Read the model definition and answer for the solid it produces. Units are mm, in the model's axes. A direction names the side the tool comes from. Coordinates: 2 decimals unless noted, no trailing zeros. Order: outer loops, then holes, each group sorted by start corner. A loop starts at its lowest first (then second) coordinate and runs counter-clockwise, first axis right, second up. Notation, with made-up numbers: (11, 1.5) -> (23, 1.5) arc R24 ccw to (23, 30.5) -> close; hole circle Ø7 at (-18.75, -36). An arc over 180 degrees is marked (long way). Use CSV: the item, a comma, the result in double quotes.
```python
from build123d import *

# Parameters (mm, degrees)
F1_ANGLE = 180
F2_R     = 18
F2_R_2   = 4.0025
F3_DEPTH = 14
F5_R     = 12
F6_DEPTH = 1
F7_R     = 4.0025
F8_DEPTH = 11


with BuildPart() as f1:
    # F0 (on Top) → F1 (revolve)
    with BuildSketch(Plane.XY):
        with BuildLine():
            ThreePointArc((0, -18), (12.727922, -12.727922), (18, 0))
            ThreePointArc((18, 0), (12.727922, 12.727922), (0, 18))
            Line((0, 18), (0, -18))
        make_face()
    revolve(axis=Axis((0, 0, 0), (0, -1, 0)), revolution_arc=F1_ANGLE)

    # F2 (on face) → F3 (cut)
    with BuildSketch(Plane(origin=(0, 0, 0), x_dir=(1, 0, 0), z_dir=(0, 0, -1))):
        Circle(F2_R)
        Circle(F2_R_2, mode=Mode.SUBTRACT)
    extrude(amount=-F3_DEPTH, mode=Mode.SUBTRACT)

    # F5 (on offset) → F6 (join)
    with BuildSketch(Plane.XY.offset(14)):
        Circle(F5_R)
    extrude(amount=F6_DEPTH)

    # F7 (on face) → F8 (join)
    with BuildSketch(Plane(origin=(0, 0, 0), x_dir=(1, 0, 0), z_dir=(0, 0, -1))):
        Circle(F7_R)
    extrude(amount=-F8_DEPTH)


solid = f1.part
```
Item 1: Find section A-A, the plane z = 5.5. Give the vertices of the cut face in (x, y) (1 decimal).
Return value:
outline,"circle Ø8 at (0, 0)"
Item 2: Each of these flat-tipped pins is pushed along its axis until it touches: P1, Ø5, axis at x = -6, y = -3, coming from the -Z side; P2, Ø1, axis at x = 1, y = 8.5, coming from the +Z side; P3, Ø4, axis at y = -2.5, z = 9.5, coming from the +X side. Where does it stop, or does it pass through?
Return value:
P1,"stops at z = 14"
P2,"stops at z = 16.1"
P3,"stops at x = 3.97"
Item 3: Straight lines are drawn through the part: line 1 along Z through (x, y) = (3.75, 10.5); line 2 along Z through (x, y) = (1.75, -0.25); line 3 along X through (y, z) = (0.5, 9.25). For each, find the intervals that lie inside material, in ascending order.
Return value:
line 1,"z = 14 to 15"
line 2,"z = 0 to 17.91"
line 3,"x = -3.97 to 3.97"
Item 4: A tool of negligible diameter and unlimited length cuts with its end or side. For faces 1 (the flat face through (-5, 9, 15)), 2 (the flat face through (0, 0, 0)), 3 (the flat face through (-3, 3, 14)), from which of +Z, -Z, +X, -X, +Y, -Y can it reach the whole face along a straight path? Write none if from no direction.
Return value:
face 1,"+Z"
face 2,"-Z, +X, -X, +Y, -Y"
face 3,"-Z"
